Read the model definition and answer for the solid it produces. Units are mm, in the model's axes. A direction names the side the tool comes from. Give positions to 0.01 mm unless a question says otherwise; leave off trailing zeros. Loops run counter-clockwise (first coordinate to the right, second up) from the corner with the lowest first, then second, coordinate; pieces in that order, holes last.
(1) Find section A-A, the plane y = 0. Write down the section's boundary in (x, z).
(2) Each of these flat-tipped pins is pushed along its axis until it touches: P1, Ø1.6, axis at x = 9.5, z = -26.5, coming from the +Y side; P2, Ø8, axis at y = 20.5, z = 21, coming from the +X side; P3, Ø5, axis at y = 22.5, z = 25, coming from the -X side. Where does it stop, or does it pass through?
(3) Determine the mould class of faces 1 (the face through (0, 7, 0)), 2 (the face through (5, 28.092, 0)), 3 (the face through (9.288, -21.015, 22.944)), 4 (the face through (3.53, 27.65, -19.45)) for opening direction Y: pulls with the +Y half, pulls with the -Y half, needs draft (parallel to the pull), parting line crosses it, or undercut.
(4) Which of the six approach directions +Z, -Z, +X, -X, +Y, -Y give full straight-line access (tool end or side, diameter ignored) to faces 5 (the face through (4.34, -14.366, -26.43)), 6 (the face through (8.56, -14, 25)), 7 (the face through (10, 18.719, -27)), 8 (the face through (3.53, -19.65, 19.8)), 9 (the face through (3.53, -27.67, -19.44))?
(5) Find section C-C, the plane x = 1.5. Write down the section's boundary in (y, z) (3 decimals).
(6) Find section D-D, the plane z = -17.5. Write down the section's boundary in (x, y), then the cut area to 3 significant figures.
(7) Straight lines are drawn through the part: probe 1 along Y at (x, z) = (8.75, 0); probe 2 along Z at (x, y) = (11, -25.5); probe 3 along Z at (x, y) = (6.25, -16.5). For each, find the intervals that lie inside material, in ascending order.
```python
from build123d import *

# Parameters (mm, degrees)
SKETCH1_W           = 56.1848
SKETCH1_H           = 56.1848
BOSS_EXTRUDE1_DEPTH = 11.3538
SKETCH2_R           = 2.54
CUT_EXTRUDE1_DEPTH  = 42.31918017
CUT_EXTRUDE2_DEPTH  = 2.794
SKETCH4_R           = 1.397
CUT_EXTRUDE3_DEPTH  = 41.640325436
FILLET1_R           = 3.175
SKETCH5_R           = 19.05
BOSS_EXTRUDE2_DEPTH = 1.5748
SKETCH6_R           = 5.3594
CUT_EXTRUDE4_DEPTH  = 42.779355829
FILLET3_R           = 0.762
SKETCH7_R           = 5.334
CUT_EXTRUDE5_DEPTH  = 7.1628
FILLET4_R           = 0.762


with BuildPart() as part:
    # Sketch1 → Boss-Extrude1 (new body)
    with BuildSketch(Plane(origin=(0, 0, 0), x_dir=(0, 0, -1), z_dir=(1, 0, 0))):
        Rectangle(SKETCH1_W, SKETCH1_H)
    extrude(amount=BOSS_EXTRUDE1_DEPTH)

    # Sketch2 → Cut-Extrude1 (cut, through all)
    with BuildSketch(Plane(origin=(11.3538, 0, 0), x_dir=(0, 0, -1), z_dir=(1, 0, 0))):
        with Locations((-23.495, 23.495)):
            Circle(SKETCH2_R)
        with Locations(Location((23.495, 23.495, 0), (0, 0, 180))):
            Circle(SKETCH2_R)
        with Locations((23.495, -23.495)):
            Circle(SKETCH2_R)
        with Locations(Location((-23.495, -23.495, 0), (0, 0, 180))):
            Circle(SKETCH2_R)
    extrude(amount=-CUT_EXTRUDE1_DEPTH, mode=Mode.SUBTRACT)

    # Sketch3 → Cut-Extrude2 (cut)
    with BuildSketch(Plane(origin=(11.3538, 0, 0), x_dir=(0, 0, -1), z_dir=(1, 0, 0))):
        with BuildLine():
            Line((-25.6794, 18.719299782), (-28.0924, 18.719299782))
            Line((-28.0924, 18.719299782), (-28.0924, 12.369299782))
            Line((-28.0924, 12.369299782), (-25.6794, 12.369299782))
            ThreePointArc((-25.6794, 12.369299782), (-22.5044, 15.544299782), (-25.6794, 18.719299782))
        make_face()
        with BuildLine():
            Line((-28.0924, -18.719299782), (-28.0924, -12.369299782))
            Line((-28.0924, -12.369299782), (-25.6794, -12.369299782))
            ThreePointArc((-25.6794, -12.369299782), (-22.5044, -15.544299782), (-25.6794, -18.719299782))
            Line((-25.6794, -18.719299782), (-28.0924, -18.719299782))
        make_face()
        with BuildLine():
            Line((28.0924, 18.719299782), (28.0924, 12.369299782))
            Line((28.0924, 12.369299782), (25.6794, 12.369299782))
            ThreePointArc((25.6794, 12.369299782), (22.5044, 15.544299782), (25.6794, 18.719299782))
            Line((25.6794, 18.719299782), (28.0924, 18.719299782))
        make_face()
        with BuildLine():
            Line((25.6794, -18.719299782), (28.0924, -18.719299782))
            Line((28.0924, -18.719299782), (28.0924, -12.369299782))
            Line((28.0924, -12.369299782), (25.6794, -12.369299782))
            ThreePointArc((25.6794, -12.369299782), (22.5044, -15.544299782), (25.6794, -18.719299782))
        make_face()
    extrude(amount=-CUT_EXTRUDE2_DEPTH, mode=Mode.SUBTRACT)

    # Sketch4 → Cut-Extrude3 (cut, through all)
    with BuildSketch(Plane(origin=(8.5598, 0, 0), x_dir=(0, 0, -1), z_dir=(1, 0, 0))):
        with Locations((-25.6794, 15.544299782)):
            Circle(SKETCH4_R)
        with Locations(Location((25.6794, 15.544299782, 0), (0, 0, 180))):
            Circle(SKETCH4_R)
        with Locations((25.6794, -15.544299782)):
            Circle(SKETCH4_R)
        with Locations(Location((-25.6794, -15.544299782, 0), (0, 0, 180))):
            Circle(SKETCH4_R)
    extrude(amount=-CUT_EXTRUDE3_DEPTH, mode=Mode.SUBTRACT)

    # Fillet1
    fillet1_edges = [part.edges().sort_by_distance(p)[0] for p in [
        (5.6769, -28.0924, -28.0924),
        (5.6769, -28.0924, 28.0924),
        (5.6769, 28.0924, 28.0924),
        (5.6769, 28.0924, -28.0924),
    ]]
    fillet(fillet1_edges, radius=FILLET1_R)

    # Sketch5 → Boss-Extrude2 (add)
    with BuildSketch(Plane(origin=(11.3538, 0, 0), x_dir=(0, 0, -1), z_dir=(1, 0, 0))):
        with Locations(Location((0, 0, 0), (0, 0, 180))):
            Circle(SKETCH5_R)
    extrude(amount=BOSS_EXTRUDE2_DEPTH)

    # Sketch6 → Cut-Extrude4 (cut, through all)
    with BuildSketch(Plane(origin=(12.9286, 0, 0), x_dir=(0, 0, -1), z_dir=(1, 0, 0))):
        Circle(SKETCH6_R)
    extrude(amount=-CUT_EXTRUDE4_DEPTH, mode=Mode.SUBTRACT)

    # Fillet3
    fillet3_edges = [part.edges().sort_by_distance(p)[0] for p in [
        (11.3538, -28.0924, 0),
        (11.3538, 21.818349891, 28.0924),
        (11.3538, 28.0924, 0),
        (11.3538, -21.818349891, -28.0924),
        (11.3538, 27.16246403, 27.16246403),
        (11.3538, 27.16246403, -27.16246403),
        (11.3538, -27.16246403, -27.16246403),
        (11.3538, -27.16246403, 27.16246403),
        (11.3538, 0, 28.0924),
        (11.3538, 15.544299782, 22.5044),
        (11.3538, 18.719299782, 26.8859),
        (11.3538, 12.369299782, 26.8859),
        (11.3538, -21.818349891, 28.0924),
        (11.3538, 0, -28.0924),
        (11.3538, 21.818349891, -28.0924),
        (11.3538, 15.544299782, -22.5044),
        (11.3538, 12.369299782, -26.8859),
        (11.3538, 18.719299782, -26.8859),
        (11.3538, -15.544299782, 22.5044),
        (11.3538, -12.369299782, 26.8859),
        (11.3538, -18.719299782, 26.8859),
        (11.3538, -15.544299782, -22.5044),
        (11.3538, -18.719299782, -26.8859),
        (11.3538, -12.369299782, -26.8859),
    ]]
    fillet(fillet3_edges, radius=FILLET3_R)

    # Sketch7 → Cut-Extrude5 (cut)
    with BuildSketch(Plane.ZY):
        with Locations((-23.495, 23.495)):
            Circle(SKETCH7_R)
        with Locations((23.495, 23.495)):
            Circle(SKETCH7_R)
        with Locations((23.495, -23.495)):
            Circle(SKETCH7_R)
        with Locations((-23.495, -23.495)):
            Circle(SKETCH7_R)
    extrude(amount=-CUT_EXTRUDE5_DEPTH, mode=Mode.SUBTRACT)

    # Fillet4
    fillet4_edges = [part.edges().sort_by_distance(p)[0] for p in [
        (3.5814, 20.790287586, -28.0924),
        (3.5814, 28.0924, -20.790287586),
        (3.5814, 28.0924, 20.790287586),
        (3.5814, 20.790287586, 28.0924),
        (3.5814, -20.790287586, 28.0924),
        (3.5814, -28.0924, 20.790287586),
        (3.5814, -20.790287586, -28.0924),
        (3.5814, -28.0924, -20.790287586),
    ]]
    fillet(fillet4_edges, radius=FILLET4_R)


solid = part.part
```
Entries:
1. outline: (0, -28.09) - (10.59, -28.09) arc R0.76 ccw to (11.35, -27.33) - (11.35, -19.05) - (12.93, -19.05) - (12.93, -5.36) - (0, -5.36) - close; (0, 5.36) - (12.93, 5.36) - (12.93, 19.05) - (11.35, 19.05) - (11.35, 27.33) arc R0.76 ccw to (10.59, 28.09) - (0, 28.09) - close
2. P1: stops at y = 27.99
2. P2: stops at x = 11.35
2. P3: stops at x = 7.16
3. face 1: needs draft
3. face 2: pulls with the +Y half
3. face 3: undercut
3. face 4: undercut
4. face 5: +X, -X
4. face 6: +Z, +X
4. face 7: -Z, +X
4. face 8: -X
4. face 9: -Z, -X
5. outline: (-28.092, -18.757) arc R0.762 ccw to (-26.851, -19.349) arc R5.334 cw to (-19.349, -26.851) arc R0.762 ccw to (-18.757, -28.092) - (18.757, -28.092) arc R0.762 ccw to (19.349, -26.851) arc R5.334 cw to (26.851, -19.349) arc R0.762 ccw to (28.092, -18.757) - (28.092, 18.757) arc R0.762 ccw to (26.851, 19.349) arc R5.334 cw to (19.349, 26.851) arc R0.762 ccw to (18.757, 28.092) - (-18.757, 28.092) arc R0.762 ccw to (-19.349, 26.851) arc R5.334 cw to (-26.851, 19.349) arc R0.762 ccw to (-28.092, 18.757) - close; hole circle Ø2.794 at (-15.544, -25.679); hole circle Ø2.794 at (-15.544, 25.679); hole circle Ø10.719 at (0, 0); hole circle Ø2.794 at (15.544, -25.679); hole circle Ø2.794 at (15.544, 25.679)
6. outline: (0, -28.09) - (10.59, -28.09) arc R0.76 ccw to (11.35, -27.33) - (11.35, -7.53) - (12.93, -7.53) - (12.93, 7.53) - (11.35, 7.53) - (11.35, 27.33) arc R0.76 ccw to (10.59, 28.09) - (0, 28.09) - close
6. area: 661 mm2
7. probe 1: y = -28.09 to -5.36, 5.36 to 28.09
7. probe 2: z = -27.92 to -25.05, -21.94 to 21.94, 25.05 to 27.92
7. probe 3: z = -28.09 to -26.7, -24.66 to 24.66, 26.7 to 28.09
